```python
from build123d import *

# Parameters (mm, degrees)
SKETCH2_R           = 3
BOSS_EXTRUDE1_DEPTH = 5
BOSS_EXTRUDE3_DEPTH = 5
CUT_EXTRUDE5_DEPTH  = 6
SKETCH10_R          = 4
SKETCH10_R_2        = 2.5
CUT_EXTRUDE6_DEPTH  = 10


with BuildPart() as part:
    # Sketch2 → Boss-Extrude1 (new body)
    with BuildSketch(Plane.XY):
        with BuildLine():
            Line((-15.626230545, 37.212307607), (-21.883589858, 37.212307607))
            ThreePointArc((-21.883589858, 37.212307607), (-24.004910201, 36.33362795), (-24.883589858, 34.212307607))
            Line((-24.883589858, 34.212307607), (-24.883589858, 14.954948294))
            ThreePointArc((-24.883589858, 14.954948294), (-24.655228455, 13.806897997), (-24.004910201, 12.83362795))
            Line((-24.004910201, 12.83362795), (-15.762269514, 4.590987263))
            ThreePointArc((-15.762269514, 4.590987263), (-15.11195126, 3.617717217), (-14.883589858, 2.46966692))
            Line((-14.883589858, 2.46966692), (-14.883589858, -3.045051706))
            ThreePointArc((-14.883589858, -3.045051706), (-15.11195126, -4.193102003), (-15.762269514, -5.16637205))
            Line((-15.762269514, -5.16637205), (-24.004910201, -13.409012737))
            ThreePointArc((-24.004910201, -13.409012737), (-24.655228455, -14.382282783), (-24.883589858, -15.53033308))
            Line((-24.883589858, -15.53033308), (-24.883589858, -34.787692393))
            ThreePointArc((-24.883589858, -34.787692393), (-24.004910201, -36.909012737), (-21.883589858, -37.787692393))
            Line((-21.883589858, -37.787692393), (-15.626230545, -37.787692393))
            ThreePointArc((-15.626230545, -37.787692393), (-14.478180248, -37.559330991), (-13.504910201, -36.909012737))
            Line((-13.504910201, -36.909012737), (-5.262269514, -28.66637205))
            ThreePointArc((-5.262269514, -28.66637205), (-4.288999468, -28.016053796), (-3.14094917, -27.787692393))
            Line((-3.14094917, -27.787692393), (2.373769455, -27.787692393))
            ThreePointArc((2.373769455, -27.787692393), (3.521819752, -28.016053796), (4.495089799, -28.66637205))
            Line((4.495089799, -28.66637205), (12.737730486, -36.909012737))
            ThreePointArc((12.737730486, -36.909012737), (13.711000532, -37.559330991), (14.85905083, -37.787692393))
            Line((14.85905083, -37.787692393), (21.116410142, -37.787692393))
            ThreePointArc((21.116410142, -37.787692393), (23.237730486, -36.909012737), (24.116410142, -34.787692393))
            Line((24.116410142, -34.787692393), (24.116410142, -15.340035571))
            ThreePointArc((24.116410142, -15.340035571), (23.9472951, -14.347014747), (23.459016571, -13.465950429))
            Line((23.459016571, -13.465950429), (22.773803714, -12.609434358))
            ThreePointArc((22.773803714, -12.609434358), (22.285525185, -11.728370039), (22.116410142, -10.735349215))
            Line((22.116410142, -10.735349215), (22.116410142, 10.159964429))
            ThreePointArc((22.116410142, 10.159964429), (22.285525185, 11.152985253), (22.773803714, 12.034049571))
            Line((22.773803714, 12.034049571), (23.459016571, 12.890565642))
            ThreePointArc((23.459016571, 12.890565642), (23.9472951, 13.771629961), (24.116410142, 14.764650785))
            Line((24.116410142, 14.764650785), (24.116410142, 34.212307607))
            ThreePointArc((24.116410142, 34.212307607), (23.237730486, 36.33362795), (21.116410142, 37.212307607))
            Line((21.116410142, 37.212307607), (14.85905083, 37.212307607))
            ThreePointArc((14.85905083, 37.212307607), (13.711000532, 36.983946204), (12.737730486, 36.33362795))
            Line((12.737730486, 36.33362795), (4.495089799, 28.090987263))
            ThreePointArc((4.495089799, 28.090987263), (3.521819752, 27.440669009), (2.373769455, 27.212307607))
            Line((2.373769455, 27.212307607), (-3.14094917, 27.212307607))
            ThreePointArc((-3.14094917, 27.212307607), (-4.288999468, 27.440669009), (-5.262269514, 28.090987263))
            Line((-5.262269514, 28.090987263), (-13.504910201, 36.33362795))
            ThreePointArc((-13.504910201, 36.33362795), (-14.478180248, 36.983946204), (-15.626230545, 37.212307607))
        make_face()
        with Locations((-16.883589858, -27.787692393)):
            Circle(SKETCH2_R, mode=Mode.SUBTRACT)
        with Locations((16.116410142, -27.787692393)):
            Circle(SKETCH2_R, mode=Mode.SUBTRACT)
        with Locations((16.116410142, 27.212307607)):
            Circle(SKETCH2_R, mode=Mode.SUBTRACT)
        with Locations((-16.883589858, 27.212307607)):
            Circle(SKETCH2_R, mode=Mode.SUBTRACT)
    extrude(amount=BOSS_EXTRUDE1_DEPTH)

    # Sketch7 → Boss-Extrude3 (add, through all)
    with BuildSketch(Plane(origin=(0, 0, 0), x_dir=(-1, 0, 0), z_dir=(0, 0, -1))):
        with BuildLine():
            Line((-24.116410142, 34.488479196), (-29.116410142, 34.488479196))
            ThreePointArc((-29.116410142, 34.488479196), (-32.651944048, 33.024013102), (-34.116410142, 29.488479196))
            Line((-34.116410142, 29.488479196), (-34.116410142, 19.488479196))
            ThreePointArc((-34.116410142, 19.488479196), (-32.651944048, 15.95294529), (-29.116410142, 14.488479196))
            Line((-29.116410142, 14.488479196), (-24.116410142, 14.488479196))
            Line((-24.116410142, 14.488479196), (-24.116410142, 34.488479196))
        make_face()
    extrude(amount=-BOSS_EXTRUDE3_DEPTH)

    # Sketch9 → Cut-Extrude5 (cut, through all)
    with BuildSketch(Plane(origin=(0, 0, 0), x_dir=(-1, 0, 0), z_dir=(0, 0, -1))):
        with BuildLine():
            Line((-24.116410142, 34.488479196), (-24.116410142, 14.488479196))
            Line((-24.116410142, 14.488479196), (-29.116410142, 14.488479196))
            ThreePointArc((-29.116410142, 14.488479196), (-32.651944048, 15.95294529), (-34.116410142, 19.488479196))
            Line((-34.116410142, 19.488479196), (-34.116410142, 29.488479196))
            ThreePointArc((-34.116410142, 29.488479196), (-32.651944048, 33.024013102), (-29.116410142, 34.488479196))
            Line((-29.116410142, 34.488479196), (-24.116410142, 34.488479196))
        make_face()
    extrude(amount=-CUT_EXTRUDE5_DEPTH, mode=Mode.SUBTRACT)

    # Sketch10 → Cut-Extrude6 (cut)
    with BuildSketch(Plane.XY.offset(5)):
        with Locations((0, 17.25)):
            Circle(SKETCH10_R)
        with Locations((0, -17.25)):
            Circle(SKETCH10_R)
        with Locations((16.5, 20)):
            Circle(SKETCH10_R_2)
        with Locations((16.5, -20)):
            Circle(SKETCH10_R_2)
        with Locations((-16.5, -20)):
            Circle(SKETCH10_R_2)
        with Locations((-16.5, 20)):
            Circle(SKETCH10_R_2)
    extrude(amount=-CUT_EXTRUDE6_DEPTH, mode=Mode.SUBTRACT)


solid = part.part
```
Could you check a few things on this model? Use its own coordinates, in mm. A direction names the side the tool comes from. Give positions to 0.01 mm unless a question says otherwise; leave off trailing zeros. Order: outer loops, then holes, each group sorted by start corner. A loop starts at its lowest first (then second) coordinate and runs counter-clockwise, first axis right, second up.
Q1. Suppose I cut it at B-B, the plane y = 16. Write out the boundary of the cut face in (x, z).
Q2. Suppose I cut it at A-A, the plane x = 0. Write out the boundary of the cut face in (y, z), and give its area (3 significant figures).
Q3. We'd pull the mould along Y, two halves only. Please class faces 1 (the flat face through (-24.884, 25, 2)), 2 (the flat face through (8.56, -32.73, 2.46)), 3 (the flat face through (-19.94, 8.77, 2.46)): +Y half, -Y half, draft (parallel to the pull), parting line (faces both ways), or undercut.
Q4. Suppose I cut it at D-D, the plane x = -16.5. Write out the boundary of the cut face in (y, z), and give its area (3 significant figures).
Q5. I'm going to push flat-ended pins straight in: P1, Ø8, axis at x = -16.88, y = 27.21, coming from the +Z side; P2, Ø3, axis at x = 16.5, y = 20, coming from the +Z side; P3, Ø1.5, axis at y = 0, z = 1.5, coming from the +X side; P4, Ø2, axis at x = 5.5, z = 3, coming from the +Y side. Where does each tip first touch, or does it pass through?
Q6. If I drill on line 1 along Y through (x, z) = (0, 1.15); line 2 along Y through (x, z) = (-16.5, 3.45); line 3 along X through (y, z) = (24.5, 4.1), over which ranges is the centre line in solid material (lowest first)?
Q7. Suppose I cut it at C-C, the plane x = 16.5. Write out the boundary of the cut face in (y, z), and give its area (3 significant figures).
Q8. For faces 4 (the cylindrical face through (13.736, -29.613, 2.465)), 5 (the flat face through (-9.326, 32.155, 2.465)), 6 (the cylindrical face through (3.51, -28.01, 2.46)), 7 (the cylindrical face through (23.943, 13.758, 2.465)), which set-ups out of +Z, -Z, +X, -X, +Y, -Y let a thin tool reach every point of the face, with its end or its side?
Solution:
1. outline: (-24.88, 0) - (-3.8, 0) - (-3.8, 5) - (-24.88, 5) - close; (3.8, 0) - (24.12, 0) - (24.12, 5) - (3.8, 5) - close
2. outline: (-27.79, 0) - (-21.25, 0) - (-21.25, 5) - (-27.79, 5) - close; (-13.25, 0) - (13.25, 0) - (13.25, 5) - (-13.25, 5) - close; (21.25, 0) - (27.21, 0) - (27.21, 5) - (21.25, 5) - close
2. area: 195 mm2
3. face 1: draft
3. face 2: -Y half
3. face 3: undercut
4. outline: (-37.79, 0) - (-30.76, 0) - (-30.76, 5) - (-37.79, 5) - close; (-24.81, 0) - (-22.5, 0) - (-22.5, 5) - (-24.81, 5) - close; (-17.5, 0) - (-5.9, 0) - (-5.9, 5) - (-17.5, 5) - close; (5.33, 0) - (17.5, 0) - (17.5, 5) - (5.33, 5) - close; (22.5, 0) - (24.24, 0) - (24.24, 5) - (22.5, 5) - close; (30.19, 0) - (37.21, 0) - (37.21, 5) - (30.19, 5) - close
4. area: 209 mm2
5. P1: stops at z = 5
5. P2: passes through
5. P3: stops at x = 22.12
5. P4: stops at y = 30.1
6. line 1: y = -27.79 to -21.25, -13.25 to 13.25, 21.25 to 27.21
6. line 2: y = -37.79 to -30.76, -24.81 to -22.5, -17.5 to -5.9, 5.33 to 17.5, 22.5 to 24.24, 30.19 to 37.21
6. line 3: x = -24.88 to -18.17, -15.6 to 14.83, 17.4 to 24.12
7. outline: (-37.79, 0) - (-30.76, 0) - (-30.76, 5) - (-37.79, 5) - close; (-24.81, 0) - (-22.5, 0) - (-22.5, 5) - (-24.81, 5) - close; (-17.5, 0) - (17.5, 0) - (17.5, 5) - (-17.5, 5) - close; (22.5, 0) - (24.24, 0) - (24.24, 5) - (22.5, 5) - close; (30.19, 0) - (37.21, 0) - (37.21, 5) - (30.19, 5) - close
7. area: 265 mm2
8. face 4: +Z, -Z
8. face 5: +Z, -Z, +Y
8. face 6: +Z, -Z, -Y
8. face 7: +Z, -Z, +X
